Here's how the part is built. I have some questions about the finished solid (model axes, mm). A direction names the side the tool comes from. Coordinates: 2 decimals unless noted, no trailing zeros. Loops run counter-clockwise (first coordinate to the right, second up) from the corner with the lowest first, then second, coordinate; pieces in that order, holes last.
Autodesk Inventor part; units mm, degrees
ref_plane "YZ Plane" through (0, 0, 0) normal (1, 0, 0) x (0, 1, 0)
ref_plane "XZ Plane" through (0, 0, 0) normal (0, 1, 0) x (-1, 0, 0)
ref_plane "XY Plane" through (0, 0, 0) normal (0, 0, 1) x (1, 0, 0)
ref_plane "Work Plane1" through (0, 0, 0) normal (0, 0, 1) x (1, 0, 0)
sketch "Sketch1" plane through (0, 0, 0) normal (0, 0, 1) x (1, 0, 0)
  circle A0 centre (0, 0) radius 25.9979
  circle A1 centre (-9.4998, -11.0022) radius 2.6601
  circle A2 centre (0.0001, -0.0022) radius 3.8801
  circle A3 centre (0.0001, -0.0022) radius 6.7754
  line L0 (10.5001, -12.5022) -> (-10.4999, -12.5022)
  line L1 (-12.4999, -10.5022) -> (-12.4999, 10.4978)
  line L2 (-10.4999, 12.4978) -> (10.5001, 12.4978)
  line L3 (12.5001, 10.4978) -> (12.5001, -10.5022)
  line L4 (12.5001, -12.5022) -> (-12.4999, 12.4978) construction
  line L5 (-12.4999, -12.5022) -> (12.5001, 12.4978) construction
  arc A4 (-10.4999, 12.4978) -> (-12.4999, 10.4978) centre (-10.4999, 10.4978) ccw
  arc A5 (-12.4999, -10.5022) -> (-10.4999, -12.5022) centre (-10.4999, -10.5022) ccw
  arc A6 (10.5001, -12.5022) -> (12.5001, -10.5022) centre (10.5001, -10.5022) ccw
  arc A7 (12.5001, 10.4978) -> (10.5001, 12.4978) centre (10.5001, 10.4978) ccw
  point P0 (0, 0)
  point P1 (-7.3029, -12.5022)
  point P2 (-12.0467, -11.77)
  dimension "d17" = 25
  dimension "d18" = 25
  dimension "d19" = 2
extrude "Extrusion1" add sketch "Sketch1" along normal blind 4 contours A0
sketch "Skizze4" plane through (0, 0, 4) normal (0, 0, 1) x (1, 0, 0)
  spline S0 degree 2 poles (24.1427, 2.2394) (24.731, 1.8489) (25.3785, 0.5587) (25.3785, -0.3311) knots 0 0 0 1 2 2 2 construction
  spline S1 degree 2 poles (25.3785, -0.3311) (25.3785, -1.1665) (24.7013, -2.5111) (24.1328, -2.8867) knots 0 0 0 1 2 2 2 construction
  spline S2 degree 2 poles (24.1328, -2.8867) (23.6682, -3.1784) (22.7141, -3.3761) (21.9726, -3.3761) knots 0 0 0 1 2 2 2 construction
  line L0 (21.9726, -3.3761) -> (20.5687, -3.3761) construction
  line L1 (20.5687, -3.3761) -> (20.5687, 2.7239) construction
  line L2 (20.5687, 2.7239) -> (21.9578, 2.7239) construction
  spline S3 degree 2 poles (21.9578, 2.7239) (22.8179, 2.7239) (23.7967, 2.4668) (24.1427, 2.2394) knots 0 0 0 1 2 2 2 construction
  spline S4 degree 2 poles (19.1896, -2.9312) (18.8979, -3.1982) (18.1564, -3.4849) (17.5978, -3.4849) knots 0 0 0 1 2 2 2 construction
  spline S5 degree 2 poles (17.5978, -3.4849) (16.9354, -3.4849) (16.0061, -3.2081) (15.5958, -3.0103) knots 0 0 0 1 2 2 2 construction
  line L3 (15.5958, -3.0103) -> (15.5958, -1.992) construction
  line L4 (15.5958, -1.992) -> (15.6551, -1.992) construction
  spline S6 degree 2 poles (15.6551, -1.992) (16.0555, -2.3677) (17.0689, -2.7829) (17.5385, -2.7829) knots 0 0 0 1 2 2 2 construction
  spline S7 degree 2 poles (17.5385, -2.7829) (18.2108, -2.7829) (18.8979, -2.2243) (18.8979, -1.7646) knots 0 0 0 1 2 2 2 construction
  spline S8 degree 2 poles (18.8979, -1.7646) (18.8979, -1.3988) (18.5371, -0.944) (18.1465, -0.8303) knots 0 0 0 1 2 2 2 construction
  spline S9 degree 2 poles (18.1465, -0.8303) (17.8648, -0.7513) (17.3952, -0.6425) (17.0442, -0.5535) knots 0 0 0 1 2 2 2 construction
  spline S10 degree 2 poles (17.0442, -0.5535) (16.7278, -0.4695) (16.2285, -0.2174) (16.0358, -0.0147) knots 0 0 0 1 2 2 2 construction
  spline S11 degree 2 poles (16.0358, -0.0147) (15.8479, 0.188) (15.6403, 0.7317) (15.6403, 1.0876) knots 0 0 0 1 2 2 2 construction
  spline S12 degree 2 poles (15.6403, 1.0876) (15.6403, 1.8291) (16.797, 2.8326) (17.6918, 2.8326) knots 0 0 0 1 2 2 2 construction
  spline S13 degree 2 poles (17.6918, 2.8326) (18.2059, 2.8326) (19.1154, 2.6299) (19.5059, 2.4372) knots 0 0 0 1 2 2 2 construction
  line L5 (19.5059, 2.4372) -> (19.5059, 1.4683) construction
  line L6 (19.5059, 1.4683) -> (19.4466, 1.4683) construction
  spline S14 degree 2 poles (19.4466, 1.4683) (19.155, 1.7352) (18.2454, 2.1307) (17.7461, 2.1307) knots 0 0 0 1 2 2 2 construction
  spline S15 degree 2 poles (17.7461, 2.1307) (17.1826, 2.1307) (16.4856, 1.6017) (16.4856, 1.1717) knots 0 0 0 1 2 2 2 construction
  spline S16 degree 2 poles (16.4856, 1.1717) (16.4856, 0.7861) (16.8959, 0.3264) (17.2815, 0.2226) knots 0 0 0 1 2 2 2 construction
  spline S17 degree 2 poles (17.2815, 0.2226) (17.5385, 0.1534) (18.285, -0.0246) (18.5321, -0.0987) knots 0 0 0 1 2 2 2 construction
  spline S18 degree 2 poles (18.5321, -0.0987) (19.1599, -0.2915) (19.7432, -1.0676) (19.7432, -1.6361) knots 0 0 0 1 2 2 2 construction
  spline S19 degree 2 poles (19.7432, -1.6361) (19.7432, -1.997) (19.4516, -2.689) (19.1896, -2.9312) knots 0 0 0 1 2 2 2 construction
  circle A0 centre (-9.9998, 17.4978) radius 1.3999 construction
  circle A1 centre (10.0001, 17.4979) radius 1.4 construction
  circle A2 centre (10.0001, -17.5021) radius 1.4 construction
  circle A3 centre (-9.9998, -17.5021) radius 1.4001 construction
  arc A4 (-25.1198, 6.6998) -> (-24.1417, 5.4917) centre (-24.1417, 6.4917) ccw construction
  line L7 (-24.1417, 5.4917) -> (-17.7002, 5.4917) construction
  arc A5 (-15.7002, 3.4917) -> (-17.7002, 5.4917) centre (-17.7002, 3.4917) ccw construction
  line L8 (-15.7002, 3.4917) -> (-15.7002, -4.496) construction
  arc A6 (-17.7002, -6.496) -> (-15.7002, -4.496) centre (-17.7002, -4.496) ccw construction
  line L9 (-17.7002, -6.496) -> (-23.8502, -6.496) construction
  arc A7 (-23.8502, -6.496) -> (-24.8235, -7.7254) centre (-23.8502, -7.496) ccw construction
  arc A8 (-24.8235, -7.7254) -> (-25.1198, 6.6998) centre (0, 0) ccw construction
  circle A9 centre (-9.4998, -11.0022) radius 2.6601 construction
  circle A10 centre (-16.8291, -16.0482) radius 1.4 construction
  circle A11 centre (6.1284, 23.0202) radius 1.4 construction
  circle A12 centre (22.7119, 7.1872) radius 1.4 construction
  circle A13 centre (0.0001, -0.0022) radius 6.5 construction
  point P0 (0, 0)
hole "Bohrung1" at (6.1284, 23.0202, 4) at (22.7119, 7.1872, 4) at (-16.8291, -16.0482, 4) direction (0, 0, -1) diameter 2.8 end through all
sketch "Skizze6" plane through (0, 0, 0) normal (0, 0, -1) x (-1, 0, 0)
  circle A0 centre (-22.7119, 7.1872) radius 1.4
  circle A1 centre (-6.1284, 23.0202) radius 1.4
  circle A2 centre (16.8291, -16.0482) radius 1.4
  circle A3 centre (0, 0) radius 25.9979
  line L0 (12.4999, -10.5022) -> (12.4999, 10.4978)
  arc A4 (12.0467, -11.77) -> (12.4999, -10.5022) centre (10.4999, -10.5022) ccw
  arc A5 (7.3029, -12.5022) -> (12.0467, -11.77) centre (9.4998, -11.0022) ccw
  line L1 (-10.5001, -12.5022) -> (7.3029, -12.5022)
  arc A6 (-12.5001, -10.5022) -> (-10.5001, -12.5022) centre (-10.5001, -10.5022) ccw
  line L2 (-12.5001, 10.4978) -> (-12.5001, -10.5022)
  arc A7 (-10.5001, 12.4978) -> (-12.5001, 10.4978) centre (-10.5001, 10.4978) ccw
  line L3 (10.4999, 12.4978) -> (-10.5001, 12.4978)
  arc A8 (12.4999, 10.4978) -> (10.4999, 12.4978) centre (10.4999, 10.4978) ccw
  arc A9 (21.6334, -14.4182) -> (15.4291, -20.9245) centre (16.8291, -16.0482) ccw
  circle A10 centre (-6.1284, 23.0202) radius 1.4
  circle A11 centre (0, 0) radius 25.9979
  arc A12 (-12.1283, 22.9955) -> (-0.9103, 25.982) centre (-6.1284, 23.0202) ccw
  circle A13 centre (-22.7119, 7.1872) radius 1.4
  arc A14 (-25.912, 2.1118) -> (-22.4096, 13.1796) centre (-22.7119, 7.1872) ccw
  point P0 (0, 0)
  point P1 (-25.912, 2.1118)
  point P2 (-0.9103, 25.982)
  dimension "d20" = 6
  dimension "d21" = 6
extrude "Extrusion4" add sketch "Skizze6" along normal blind 4 contours A12 A3 | A3 A9 | A14 A3
sketch "Skizze7" plane through (0, 0, 0) normal (0, 0, -1) x (-1, 0, 0)
  arc A0 (-25.912, 2.1118) -> (-22.4096, 13.1796) centre (-22.7119, 7.1872) ccw
  arc A1 (-25.912, 2.1118) -> (15.4291, -20.9245) centre (0, 0) ccw
  arc A2 (21.6334, -14.4182) -> (15.4291, -20.9245) centre (16.8291, -16.0482) ccw
  arc A3 (21.6334, -14.4182) -> (-0.9103, 25.982) centre (0, 0) ccw
  arc A4 (-12.1283, 22.9955) -> (-0.9103, 25.982) centre (-6.1284, 23.0202) ccw
  arc A5 (-12.1283, 22.9955) -> (-22.4096, 13.1796) centre (0, 0) ccw
  line L0 (12.4999, -10.5022) -> (12.4999, 10.4978)
  arc A6 (12.0467, -11.77) -> (12.4999, -10.5022) centre (10.4999, -10.5022) ccw
  arc A7 (7.3029, -12.5022) -> (12.0467, -11.77) centre (9.4998, -11.0022) ccw
  line L1 (-10.5001, -12.5022) -> (7.3029, -12.5022)
  arc A8 (-12.5001, -10.5022) -> (-10.5001, -12.5022) centre (-10.5001, -10.5022) ccw
  line L2 (-12.5001, 10.4978) -> (-12.5001, -10.5022)
  arc A9 (-10.5001, 12.4978) -> (-12.5001, 10.4978) centre (-10.5001, 10.4978) ccw
  line L3 (10.4999, 12.4978) -> (-10.5001, 12.4978)
  arc A10 (12.4999, 10.4978) -> (10.4999, 12.4978) centre (10.4999, 10.4978) ccw
  circle A11 centre (8.3387, 18.1787) radius 4
  circle A12 centre (-0.0001, -20) radius 4
  circle A13 centre (-19.3477, -5.0663) radius 4
  circle A14 centre (0, 0) radius 20 construction
  point P0 (0, 0)
  dimension "d24" = 8
  dimension "d25" = 8
  dimension "d26" = 8
  dimension "d29" = 40
extrude "Extrusion5" cut sketch "Skizze7" against normal blind 3 contours A11 | A12 | A13
sketch "Skizze8" plane through (0, 0, -4) normal (0, 0, -1) x (-1, 0, 0)
  circle A0 centre (16.8271, -16.0472) radius 2.75
  circle A1 centre (-22.7139, 7.1882) radius 2.75
  circle A2 centre (-6.1303, 23.0212) radius 2.75
  circle A3 centre (-6.1303, 23.0212) radius 3.25
  circle A4 centre (-22.7139, 7.1882) radius 3.25
  circle A5 centre (16.8271, -16.0472) radius 3.25
  circle A6 centre (-10.002, -17.5012) radius 2.75
  circle A7 centre (9.998, -17.5011) radius 2.75
  circle A8 centre (-10.002, 17.4988) radius 2.75
  circle A9 centre (-10.002, 17.4988) radius 3.25
  circle A10 centre (-10.002, -17.5012) radius 3.25
  circle A11 centre (9.998, -17.5011) radius 3.25
  point P0 (0, 0)
  dimension "d30" = 0.5
  dimension "d31" = 0.5
  dimension "d32" = 0.5
  dimension "d33" = 0.5
  dimension "d34" = 0.5
  dimension "d35" = 0.5
extrude "Extrusion6" cut sketch "Skizze8" against normal up to surface (4 mm away) contours A6 | A7 | A8 | A9 | A10 | A11
properties part number "Anglerfish_flipped_LidMoun"
Q1. For faces 5 (the cylindrical face through (-16.506, -10.985, -1.972)), 6 (the cylindrical face through (-13.184, -16.858, -2.028)), 7 (the flat face through (21, 6, -4)), 8 (the cylindrical face through (15.532, -3.865, 1.479)), 9 (the cylindrical face through (11.93, -11.9, 1.97)), which set-ups out of +Z, -Z, +X, -X, +Y, -Y let a thin tool reach every point of the face, with its end or its side?
Q2. Will these pins go through, and if not, where does the flat tip stop? P1, Ø2, axis at y = 4, z = 3, coming from the -X side; P2, Ø6.5, axis at x = -6.5, y = 19, coming from the -Z side; P3, Ø1.2, axis at x = 5, z = 2.5, coming from the +Y side.
Q3. We'd pull the mould along Y, two halves only. Please class faces 1 (the cylindrical face through (16.95, 5.52, -1.97)), 2 (the cylindrical face through (-13.993, -20.255, -1.972)), 3 (the flat face through (4.9, 21.6, -4)), 4 (the cylindrical face through (-7.472, 14.274, 1.479)): pulls with the +Y half, pulls with the -Y half, needs draft (parallel to the pull), parting line crosses it, or undercut.
Q4. Suppose I cut it at A-A on y = 0. Write out the boundary of the cut face in (x, z), and give its area (3 significant figures).
Q5. Suppose I cut it at B-B on z = 0.75. Write out the boundary of the cut face in (x, y).
Q6. Please list where these lines run through material, in increasing order: probe 1 along Z at (x, y) = (-2.5, 16); probe 2 along X at (y, z) = (-17, -0.5); probe 3 along X at (y, z) = (-8.5, 1.5).
Q7. Suppose I cut it at C-C on y = -20. Write out the boundary of the cut face in (x, z), and give its area (3 significant figures).
Check values:
1. face 5: -Z, +Y
1. face 6: -Z, +X
1. face 7: -Z, +X, -X, +Y, -Y
1. face 8: -Z
1. face 9: +Z, -Z
2. P1: stops at x = -25.82
2. P2: stops at z = 0
2. P3: stops at y = 25.62
3. face 1: parting line crosses it
3. face 2: pulls with the -Y half
3. face 3: needs draft
3. face 4: undercut
4. outline: (-26, 0) - (-12.5, 0) - (-12.5, 4) - (-26, 4) - close; (12.5, 0) - (26, 0) - (26, 4) - (12.5, 4) - close
4. area: 108 mm2
5. outline: circle Ø52 at (0, 0); hole circle Ø2.8 at (-16.83, -16.05); hole (-12.5, -10.5) arc R2 ccw to (-12.05, -11.77) arc R2.66 ccw to (-7.3, -12.5) - (10.5, -12.5) arc R2 ccw to (12.5, -10.5) - (12.5, 10.5) arc R2 ccw to (10.5, 12.5) - (-10.5, 12.5) arc R2 ccw to (-12.5, 10.5) - close; hole circle Ø8 at (-8.34, 18.18); hole circle Ø8 at (0, -20); hole circle Ø2.8 at (6.13, 23.02); hole circle Ø8 at (19.35, -5.07); hole circle Ø2.8 at (22.71, 7.19)
6. probe 1: z = 0 to 4
6. probe 2: x = -19.67 to -17.86, -15.8 to -13.21
6. probe 3: x = -24.57 to -12.5, 12.5 to 17.3, 21.4 to 24.57
7. outline: (-16.61, -4) - (-13.65, -4) - (-13.65, 0) - (-4, 0) - (-4, 3) - (4, 3) - (4, 0) - (16.61, 0) - (16.61, 4) - (-16.61, 4) - close
7. area: 121 mm2
